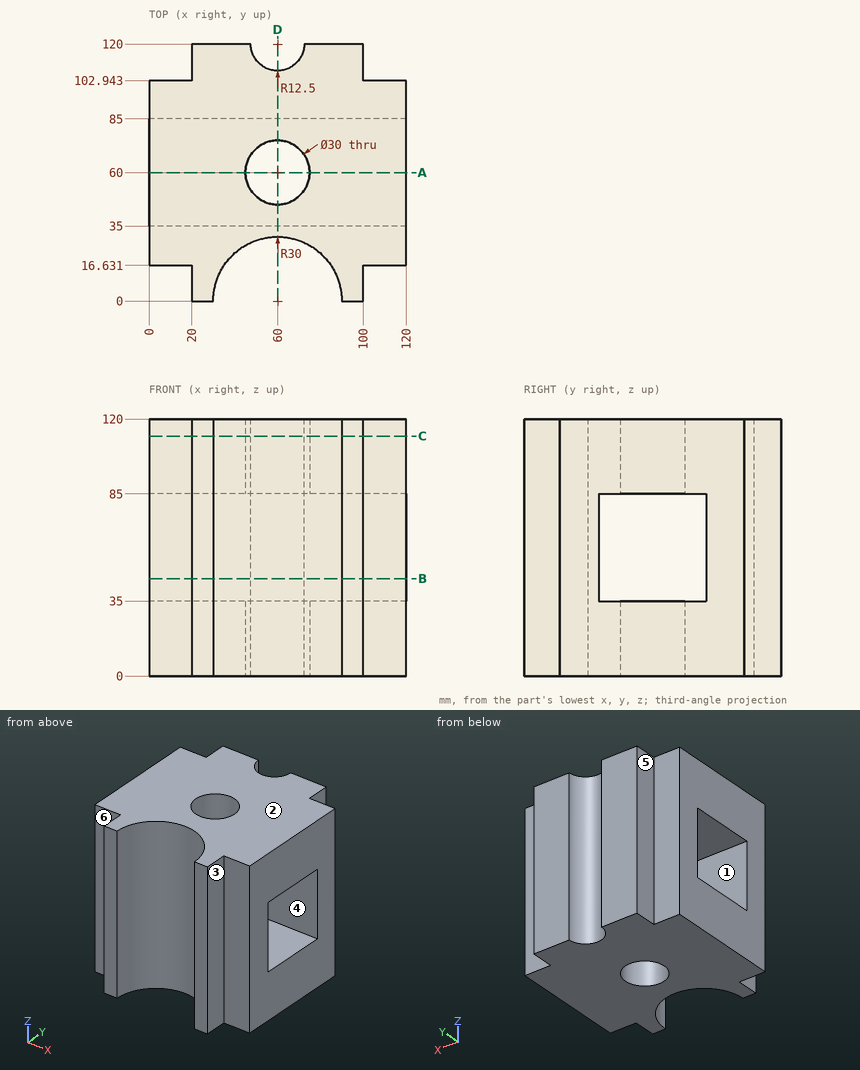
Part print with two shaded views. Sizes in mm from the minimum x, y, z corner. A direction names the side the tool comes from. Round coordinates to 2 decimals unless told otherwise and drop trailing zeros. Write each loop counter-clockwise with the first axis right and the second up, starting at its lowest first coordinate (ties: lowest second). Pieces come first, ordered by that corner, then holes. Notation, with made-up numbers: (78.5, -8) -> (108.5, -8) arc R30 cw to (108.5, 19) -> close; hole circle Ø10 at (6, -34.5). An arc over 180 degrees is marked (long way). Use one line per item in the form item = value.
Q1. Band-saw the part on B-B, the plane z = 45.5. Write the cut outline in (x, y), then the cut area to 3 significant figures.
Conclusion:
outline = (0, 16.63) -> (20, 16.63) -> (20, 0) -> (30, 0) arc R30 cw to (90, 0) -> (100, 0) -> (100, 16.63) -> (120, 16.63) -> (120, 35) -> (0, 35) -> close; (0, 85) -> (120, 85) -> (120, 102.94) -> (100, 102.94) -> (100, 120) -> (72.5, 120) arc R12.5 cw to (47.5, 120) -> (20, 120) -> (20, 102.94) -> (0, 102.94) -> close
area = 5,390 mm²
Q2. Band-saw the part on C-C, the plane z = 112. Write the cut outline in (x, y), then the cut area to 3 significant figures.
Conclusion:
outline = (0, 16.63) -> (20, 16.63) -> (20, 0) -> (30, 0) arc R30 cw to (90, 0) -> (100, 0) -> (100, 16.63) -> (120, 16.63) -> (120, 102.94) -> (100, 102.94) -> (100, 120) -> (72.5, 120) arc R12.5 cw to (47.5, 120) -> (20, 120) -> (20, 102.94) -> (0, 102.94) -> close; hole circle Ø30 at (60, 60)
area = 10,700 mm²
Q3. Two-plate mould, pull along Z, no slides. Class the marked faces 1, 2 and 3: released by +Z, released by -Z, zero draft, split by the parting line, or undercut.
Conclusion:
face_1 = undercut
face_2 = released by +Z
face_3 = zero draft
Q4. Drop flat-ended pins along their axis: P1, Ø3, axis at x = 103.5, y = 56.5, coming from the -Z side; P2, Ø10, axis at x = 11, z = 41, coming from the -Y side; P3, Ø13.5, axis at y = 113.5, z = 88, coming from the +X side; P4, Ø13.5, axis at y = 5.5, z = 53, coming from the -X side. Give the stop position or say it passes through.
Conclusion:
P1 = 0
P2 = 16.63
P3 = 100
P4 = 20
Q5. Band-saw the part on D-D, the plane x = 60. Write the cut outline in (y, z), then the cut area to 3 significant figures.
Conclusion:
outline = (30, 0) -> (45, 0) -> (45, 35) -> (35, 35) -> (35, 85) -> (45, 85) -> (45, 120) -> (30, 120) -> close; (75, 0) -> (107.5, 0) -> (107.5, 120) -> (75, 120) -> (75, 85) -> (85, 85) -> (85, 35) -> (75, 35) -> close
area = 4,700 mm²
Q6. Tool access for the marked faces 4, 5 and 6: list every direction of +Z, -Z, +X, -X, +Y, -Y with a clear straight run to the whole face (end or side of a thin tool).
Conclusion:
face_4 = +X, -X
face_5 = +Z, -Z, -X, +Y
face_6 = +Z, -Z, -X, -Y
Q7. Band-saw the part on A-A, the plane y = 60. Write the cut outline in (x, z).
Conclusion:
outline = (0, 0) -> (45, 0) -> (45, 35) -> (0, 35) -> close; (0, 85) -> (45, 85) -> (45, 120) -> (0, 120) -> close; (75, 0) -> (120, 0) -> (120, 35) -> (75, 35) -> close; (75, 85) -> (120, 85) -> (120, 120) -> (75, 120) -> close
Q8. Drill centre lines: L1, parallel to Y at x = 60, z = 93; L2, parallel to Z at x = 104.5, y = 47.5; L3, parallel to X at y = 60, z = 12. Where is each one in solid material? Low to high.
Conclusion:
L1 = 30 to 45, 75 to 107.5
L2 = 0 to 35, 85 to 120
L3 = 0 to 45, 75 to 120
